Here's how the part is built. I have some questions about the finished solid (model axes, mm). Coordinates: 2 decimals unless noted, no trailing zeros. Loops run counter-clockwise (first coordinate to the right, second up) from the corner with the lowest first, then second, coordinate; pieces in that order, holes last. Notation, with made-up numbers: M 72,42.25 L 131,42.25 A17 ccw 131,73.25 Z; hole C 52,88 d2. An arc over 180 degrees is marked long. Use CSV: the item, a comma, the result in double quotes. Start each with the question number.
Q1. If we section it at A-A (z = -5.25): Please give me the cut outline in (x, y).
Q2. If we section it at B-B (x = 34.15): Please give me the cut outline in (y, z).
Q3. Please list where these lines run through material, in increasing order: probe 1 along X at (y, z) = (11.8, 1.25); probe 2 along Y at (x, z) = (34.3, 0.5); probe 3 along X at (y, z) = (12.3, -0.5). Write a range as [from, to].
Q4. If we section it at C-C (y = 12.25): Please give me the cut outline in (x, z).
from build123d import *

# Parameters (mm, degrees)
CYLINDER_R     = 0.7
CYLINDER_DEPTH = 10


with BuildPart() as cilindro:
    # Cylinder → Cylinder (new body)
    with BuildSketch(Plane(origin=(3, 5.25, -8), x_dir=(1, 0, 0), z_dir=(0, 0, 1))):
        Circle(CYLINDER_R)
    extrude(amount=CYLINDER_DEPTH)


with BuildPart() as part_mirroring:
    # Part__Mirroring: instance of Cilindro
    add(cilindro.part.mirror(Plane(origin=(0, 0, 0), x_dir=(0, 1, 0), z_dir=(0, 0, 1))))


with BuildPart() as part_mirroring_1:
    # Part__Mirroring placement: moved
    add(part_mirroring.part.moved(Location((0, 6.5, -6))))


with BuildPart() as part_mirroring001:
    # Part__Mirroring001: instance of Part__Mirroring
    add(part_mirroring_1.part.mirror(Plane(origin=(0, 0, 0), x_dir=(0, 1, 0), z_dir=(0, 0, 1))))


with BuildPart() as part_mirroring001_1:
    # Part__Mirroring001 placement: moved
    add(part_mirroring001.part.moved(Location((31, 0, -6))))


solid = part_mirroring001_1.part
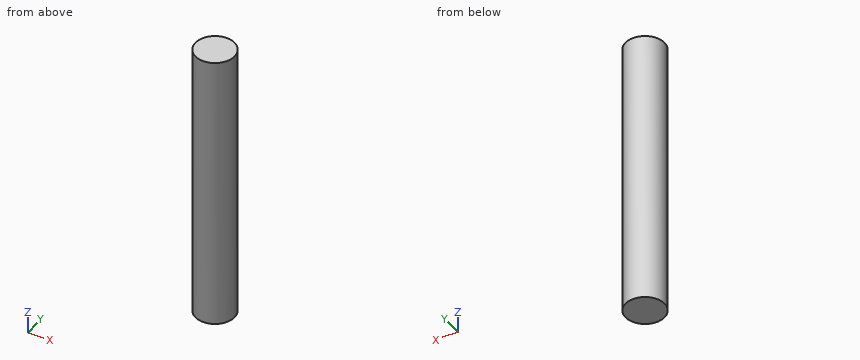
Results below:
1,outline,"C 34,11.75 d1.4"
2,outline,"M 11.07,-8 L 12.43,-8 L 12.43,2 L 11.07,2 Z"
3,probe 1,"[33.3, 34.7]"
3,probe 2,"[11.12, 12.38]"
3,probe 3,"[33.57, 34.43]"
4,outline,"M 33.51,-8 L 34.49,-8 L 34.49,2 L 33.51,2 Z"
